from build123d import *

# Parameters (mm, degrees)
SKETCH2_R           = 42
BOSS_EXTRUDE1_DEPTH = 11.5
SKETCH3_R           = 8
CUT_EXTRUDE1_DEPTH  = 7


with BuildPart() as part:
    # Sketch2 → Boss-Extrude1 (new body)
    with BuildSketch(Plane(origin=(0, 0, 0), x_dir=(1, 0, 0), z_dir=(0, 1, 0))):
        with Locations(Location((0, 0, 0), (0, 0, 270))):
            Circle(SKETCH2_R)
        Polygon((0, 7.505553499), (-6.5, 3.75277675), (-6.5, -3.75277675), (0, -7.505553499), (6.5, -3.75277675), (6.5, 3.75277675), align=None, mode=Mode.SUBTRACT)
    extrude(amount=BOSS_EXTRUDE1_DEPTH)

    # Sketch3 → Cut-Extrude1 (cut)
    with BuildSketch(Plane.XZ):
        with Locations(Location((0, 0, 0), (0, 0, 270))):
            Circle(SKETCH3_R)
    extrude(amount=-CUT_EXTRUDE1_DEPTH, mode=Mode.SUBTRACT)

    # Sketch4 → Revolve1 (revolve)
    with BuildSketch(Plane.XY, mode=Mode.PRIVATE) as revolve1_sk:
        with BuildLine():
            Line((4.05, 14.719341476), (4.05, 11.5))
            Line((4.05, 11.5), (42, 11.5))
            Line((42, 11.5), (42, 52))
            Line((42, 52), (37.5, 52))
            ThreePointArc((37.5, 52), (27.911691099, 26.956288214), (4.05, 14.719341476))
        make_face()
    revolve(revolve1_sk.sketch.rotate(Axis((0, 0, 0), (0, 1, 0)), 90), axis=Axis((0, 0, 0), (0, 1, 0)))


solid = part.part
Design review of the part built by this model. Coordinates are the model's own, in mm. A direction names the side the tool comes from. Coordinates: 2 decimals unless noted, no trailing zeros. Loops run counter-clockwise (first coordinate to the right, second up) from the corner with the lowest first, then second, coordinate; pieces in that order, holes last.
Item 1: Add section B-B (y = 13.5). Write out the cut boundary in (x, z).
Completed:
outline: circle Ø84 at (0, 0); hole circle Ø8.1 at (0, 0)
Item 2: Clearance check with flat-ended pins moving along their axes: pin 1 (8 mm diameter, centred on x = -14, y = 10.5, fed in from +Z); pin 2 (1.3 mm diameter, centred on y = 10, z = 0.5, fed in from +X); pin 3 (2 mm diameter, centred on y = 10.5, z = 0, fed in from -X). State where each tip first meets the part, or that it passes through.
Completed:
pin 1: stops at z = 40.79
pin 2: stops at x = 42
pin 3: stops at x = -42
Item 3: Wall thickness on L1, parallel to X at y = 13.85, z = 0; L2, parallel to X at y = 1, z = 0; L3, parallel to Z at x = -0.5, y = 25.5: over which ranges is each line inside the solid? List them lowest first.
Completed:
L1: x = -42 to -4.05, 4.05 to 42
L2: x = -42 to -8, 8 to 42
L3: z = -42 to -26.53, 26.53 to 42
Item 4: Add section C-C (z = 21.5). Write out the cut boundary in (x, y).
Completed:
outline: (-36.08, 0) - (36.08, 0) - (36.08, 52) - (30.72, 52) arc R30.72 cw to (-30.72, 52) - (-36.08, 52) - close
Item 5: For faces 4 (the flat face through (-34.4, 52, 15.8)), 5 (the flat face through (-3.3, 9.2, 5.6)), list the 3-axis set-ups (+Z, -Z, +X, -X, +Y, -Y) from which the entire face can be reached by the end or side of a thin tool; tool diameter is ignored.
Completed:
face 4: +Z, -Z, +X, -X, +Y
face 5: -Y
Item 6: Add section D-D (x = 29). Write out the cut boundary in (y, z), and give its area (3 significant figures).
Completed:
outline: (0, -30.38) - (52, -30.38) - (52, -23.77) arc R23.77 cw to (52, 23.77) - (52, 30.38) - (0, 30.38) - close
area: 2,270 mm2
Item 7: Draft analysis for pull direction X (two halves, no side actions). For faces 1 (the cylindrical face through (-41.91, 26.36, -2.77)), 2 (the flat face through (-9, 0, -1)), 3 (the cylindrical face through (3.954, 13.087, 0.878)), state which applies: pulls with the +X half, pulls with the -X half, needs draft (parallel to the pull), parting line crosses it, or undercut.
Completed:
face 1: parting line crosses it
face 2: needs draft
face 3: undercut
Item 8: Add section A-A (z = 0). Write out the cut boundary in (x, y), and give its area (3 significant figures).
Completed:
outline: (-42, 0) - (-8, 0) - (-8, 7) - (-6.5, 7) - (-6.5, 11.5) - (-4.05, 11.5) - (-4.05, 14.72) arc R37.5 cw to (-37.5, 52) - (-42, 52) - close; (4.05, 11.5) - (6.5, 11.5) - (6.5, 7) - (8, 7) - (8, 0) - (42, 0) - (42, 52) - (37.5, 52) arc R37.5 cw to (4.05, 14.72) - close
area: 1,960 mm2
